from build123d import *

# Parameters (mm, degrees)
SKETCH1_R           = 1.125
SKETCH1_R_2         = 2
SKETCH1_W           = 5.2
SKETCH1_H           = 12.2
SKETCH1_W_2         = 5
SKETCH1_H_2         = 6.5
BOSS_EXTRUDE1_DEPTH = 3
FILLET1_R           = 1


with BuildPart() as part:
    # Sketch1 → Boss-Extrude1 (new body)
    with BuildSketch(Plane.XY):
        with BuildLine():
            Line((23.501825189, 8.05), (23.501825189, 14.369504832))
            ThreePointArc((23.501825189, 14.369504832), (21.501825189, 17.5), (23.501825189, 20.630495168))
            Line((23.501825189, 20.630495168), (23.501825189, 26.95))
            ThreePointArc((23.501825189, 26.95), (24.380504846, 29.071320344), (26.501825189, 29.95))
            Line((26.501825189, 29.95), (33.522833629, 29.95))
            ThreePointArc((33.522833629, 29.95), (35.951825189, 30.95), (38.38081675, 29.95))
            Line((38.38081675, 29.95), (45.401825189, 29.95))
            ThreePointArc((45.401825189, 29.95), (47.523145533, 29.071320344), (48.401825189, 26.95))
            Line((48.401825189, 26.95), (48.401825189, 20.630495168))
            ThreePointArc((48.401825189, 20.630495168), (50.401825189, 17.5), (48.401825189, 14.369504832))
            Line((48.401825189, 14.369504832), (48.401825189, 8.05))
            ThreePointArc((48.401825189, 8.05), (47.523145533, 5.928679656), (45.401825189, 5.05))
            Line((45.401825189, 5.05), (38.38081675, 5.05))
            ThreePointArc((38.38081675, 5.05), (35.951825189, 4.05), (33.522833629, 5.05))
            Line((33.522833629, 5.05), (26.501825189, 5.05))
            ThreePointArc((26.501825189, 5.05), (24.380504846, 5.928679656), (23.501825189, 8.05))
        make_face()
        with Locations((24.951825189, 17.5)):
            Circle(SKETCH1_R, mode=Mode.SUBTRACT)
        with Locations((46.951825189, 17.5)):
            Circle(SKETCH1_R, mode=Mode.SUBTRACT)
        with Locations((44.401825189, 11)):
            Circle(SKETCH1_R_2, mode=Mode.SUBTRACT)
        with Locations((30.551825189, 17.5)):
            Rectangle(SKETCH1_W, SKETCH1_H, mode=Mode.SUBTRACT)
        with Locations((43.901825189, 23.75)):
            Rectangle(SKETCH1_W_2, SKETCH1_H_2, mode=Mode.SUBTRACT)
    extrude(amount=BOSS_EXTRUDE1_DEPTH)

    # Fillet1
    fillet1_edges = [part.edges().sort_by_distance(p)[0] for p in [
        (35.951825189, 4.05, 3),
        (41.891320969, 5.05, 3),
        (47.523145533, 5.928679656, 3),
        (48.401825189, 11.209752416, 3),
        (50.401825189, 17.5, 3),
        (48.401825189, 23.790247584, 3),
        (47.523145533, 29.071320344, 3),
        (41.891320969, 29.95, 3),
        (35.951825189, 30.95, 3),
        (30.012329409, 29.95, 3),
        (24.380504846, 5.928679656, 3),
        (24.380504846, 29.071320344, 3),
        (23.501825189, 23.790247584, 3),
        (21.501825189, 17.5, 3),
        (23.501825189, 11.209752416, 3),
        (30.012329409, 5.05, 3),
    ]]
    fillet(fillet1_edges, radius=FILLET1_R)


solid = part.part
Input: part model. Units: mm. Frame: model coordinates. A direction names the side the tool comes from. Coordinates: 2 decimals unless noted, no trailing zeros. Write each loop counter-clockwise with the first axis right and the second up, starting at its lowest first coordinate (ties: lowest second). Pieces come first, ordered by that corner, then holes. Notation, with made-up numbers: M 19,-11.5 L 56,-11.5 A33 cw 56,24.5 Z; hole C -39.75,76.5 d5. An arc over 180 degrees is marked long. Answer as a JSON object with one key per item and string values. Group by question number.
(1) Section A-A on z = 1.05. Give the number of separate pieces and of enclosed holes in the cut face, plus the area to 3 significant figures.
(2) Contact query for flat-ended pins moving along their axis: P1, Ø0.9, axis at x = 43, z = 2, coming from the +Y side; P2, Ø1.8, axis at x = 24.95, y = 17.5, coming from the -Z side; P3, Ø0.9, axis at x = 31.5, z = 2, coming from the -Y side; P4, Ø0.6, axis at y = 23, z = 1, coming from the -X side. Output: stop coordinate, or through.
(3) Ray query, line 1 along X through (y, z) = (23.5, 0.4); line 2 along X through (y, z) = (24.75, 1.6); line 3 along X through (y, z) = (14, 1.9). Return the intervals inside material, ascending. Write a range as [from, to].
(4) Section D-D on y = 17.5. Output: boundary loops of the cut face in (x, z), plus the area to 3 significant figures.
(5) Mould query, pull axis X, two halves, no side actions, for faces 4 (the face through (47.546, 5.952, 0.986)), 5 (the face through (41.402, 24, 1)), 6 (the face through (21.502, 17.445, 0.986)), 7 (the face through (41.717, 29.665, 2.699)). Classes: pulls with the +X half, pulls with the -X half, needs draft (parallel to the pull), parting line crosses it, or undercut.
(6) Set-up query: faces 1 (the face through (42, 29.95, 1)), 2 (the face through (48.402, 11, 1)), 3 (the face through (31, 23.6, 1)). Return all of +Z, -Z, +X, -X, +Y, -Y with unobstructed straight access to the full face (end or side cutting, diameter ignored); none if empty.
(7) Section B-B on y = 11. Output: boundary loops of the cut face in (x, z), plus the area to 3 significant figures.
(8) Section C-C on x = 31.5. Output: boundary loops of the cut face in (y, z).
Result set:
{
 "1": {"separate pieces": "1", "enclosed holes": "5", "area": "521 mm2"},
 "2": {"P1": "stops at y = 29.95", "P2": "passes through", "P3": "stops at y = 5.05", "P4": "stops at x = 23.5"},
 "3": {"line 1": "x = [23.5, 27.95], [33.15, 41.4], [46.4, 48.4]", "line 2": "x = [23.5, 41.4], [46.4, 48.4]", "line 3": "x = [23.5, 27.95], [33.15, 48.4]"},
 "4": {"outline": "M 21.5,0 L 23.83,0 L 23.83,3 L 22.5,3 A1 ccw 21.5,2 Z; M 26.08,0 L 27.95,0 L 27.95,3 L 26.08,3 Z; M 33.15,0 L 45.83,0 L 45.83,3 L 33.15,3 Z; M 48.08,0 L 50.4,0 L 50.4,2 A1 ccw 49.4,3 L 48.08,3 Z", "area": "57.2 mm2"},
 "5": {"face 4": "pulls with the +X half", "face 5": "undercut", "face 6": "pulls with the -X half", "face 7": "needs draft"},
 "6": {"face 1": "+Z, -Z, +X, +Y", "face 2": "+Z, -Z, +X, -Y", "face 3": "+Z, -Z"},
 "7": {"outline": "M 23.5,0 L 42.4,0 L 42.4,3 L 24.5,3 A1 ccw 23.5,2 Z; M 46.4,0 L 48.4,0 L 48.4,2 A1 ccw 47.4,3 L 46.4,3 Z", "area": "62.3 mm2"},
 "8": {"outline": "M 5.05,0 L 11.4,0 L 11.4,3 L 6.05,3 A1 ccw 5.05,2 Z; M 23.6,0 L 29.95,0 L 29.95,2 A1 ccw 28.95,3 L 23.6,3 Z"}
}
